Study the drawing (mm; zero at the part's minimum x, y, z) and answer. A direction names the side the tool comes from. Give positions to 0.01 mm unless a question says otherwise; leave off trailing zeros. Loops run counter-clockwise (first coordinate to the right, second up) from the corner with the lowest first, then second, coordinate; pieces in that order, holes last. Notation, with made-up numbers: (66.25, -31) - (116.25, -31) arc R19 ccw to (116.25, -22) - close; hole circle Ø6 at (25.5, 44.5). An arc over 180 degrees is marked (long way). Answer in a Markdown table with one row per item. Add a question column.
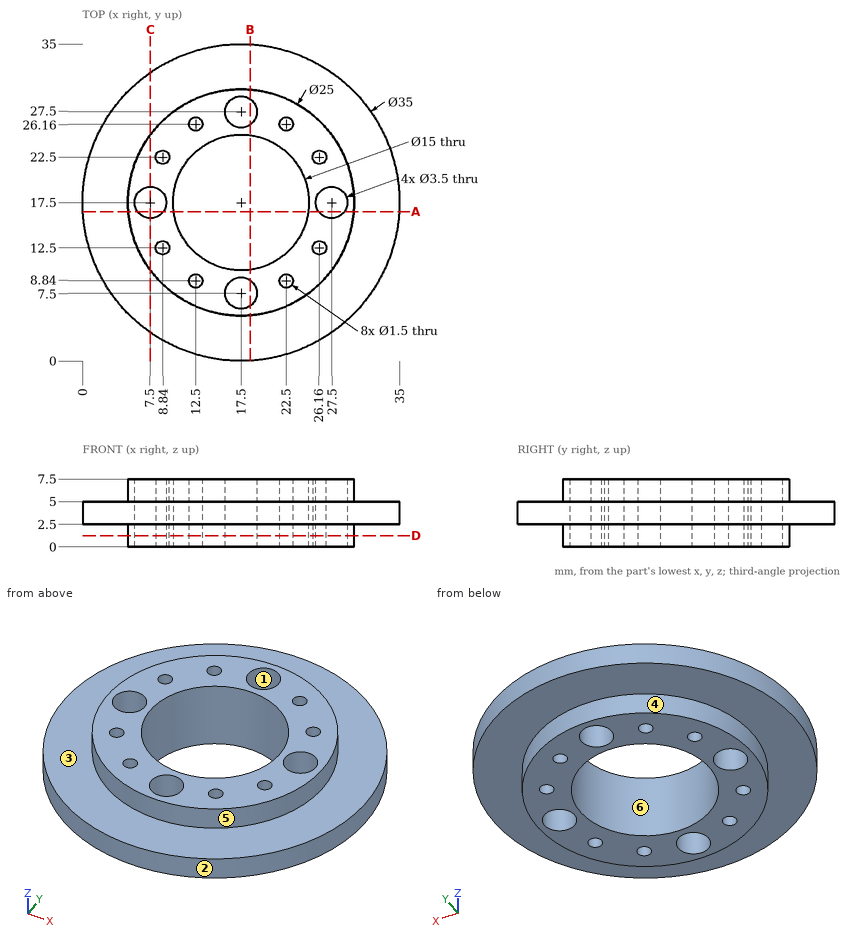
(1) Given pin 1 Ø10 at (x, y) = (4, 5) entering from -Z; pin 2 Ø2 at (y, z) = (26, 4.5) entering from -X; pin 3 Ø2 at (y, z) = (23, 4) entering from -X, each flat-ended and moving along its own axis, determine where each tip first touches the part or whether it passes through.
(2) A cutting plane is placed at C-C on x = 7.5. Determine the outline of the cut face in (y, z).
(3) A cutting plane is placed at D-D on z = 1.25. Give the number of separate pieces and of enclosed holes in the cut face.
(4) The mould has two halves that part along Y. Classify the marked faces 1, 2 and 3: pulls with the +Y half, pulls with the -Y half, needs draft (parallel to the pull), parting line crosses it, or undercut.
(5) Find the intervals of material crossed by line 1 along Y through (x, z) = (17.5, 2.25); line 2 along Y through (x, z) = (12.5, 4.5); line 3 along X through (y, z) = (18, 1.25), in increasing order. Write a range as [from, to].
(6) A tool of negligible diameter and unlimited length cuts with its end or side. For the marked faces 4, 5 and 6, from which of +Z, -Z, +X, -X, +Y, -Y can it reach the whole face along a straight path? Write none if from no direction.
(7) A cutting plane is placed at A-A on y = 16.5. Determine the outline of the cut face in (x, z).
Evaluation:
| question | item | result |
|---|---|---|
| 1 | pin 1 | stops at z = 2.5 |
| 1 | pin 2 | stops at x = 1.69 |
| 1 | pin 3 | stops at x = 0.59 |
| 2 | outline | (3.14, 2.5) - (10, 2.5) - (10, 0) - (15.75, 0) - (15.75, 7.5) - (10, 7.5) - (10, 5) - (3.14, 5) - close; (19.25, 0) - (25, 0) - (25, 2.5) - (31.86, 2.5) - (31.86, 5) - (25, 5) - (25, 7.5) - (19.25, 7.5) - close |
| 3 | separate pieces | 1 |
| 3 | enclosed holes | 13 |
| 4 | face 1 | undercut |
| 4 | face 2 | parting line crosses it |
| 4 | face 3 | needs draft |
| 5 | line 1 | y = [5, 5.75], [9.25, 10], [25, 25.75], [29.25, 30] |
| 5 | line 2 | y = [0.73, 8.09], [9.59, 11.91], [23.09, 25.41], [26.91, 34.27] |
| 5 | line 3 | x = [5.01, 5.82], [9.18, 10.02], [24.98, 25.82], [29.18, 29.99] |
| 6 | face 4 | -Z |
| 6 | face 5 | +Z |
| 6 | face 6 | +Z, -Z |
| 7 | outline | (0.03, 2.5) - (5.04, 2.5) - (5.04, 0) - (6.06, 0) - (6.06, 7.5) - (5.04, 7.5) - (5.04, 5) - (0.03, 5) - close; (8.94, 0) - (10.07, 0) - (10.07, 7.5) - (8.94, 7.5) - close; (24.93, 0) - (26.06, 0) - (26.06, 7.5) - (24.93, 7.5) - close; (28.94, 0) - (29.96, 0) - (29.96, 2.5) - (34.97, 2.5) - (34.97, 5) - (29.96, 5) - (29.96, 7.5) - (28.94, 7.5) - close |
